from build123d import *

# Parameters (mm, degrees)
SKETCH_1_R               = 15.5
EXTRUDE_1_DEPTH          = 10
SKETCH_2_W               = 1.7
SKETCH_2_H               = 2.2
SKETCH_4_R               = 11.5
CUT_EXTRUDE_1_DEPTH      = 14
SKETCH_5_R               = 5.25
CUT_EXTRUDE_2_DEPTH      = 15
CHAMFER_1_SIZE           = 2
CUT_EXTRUDE_START        = -2
SKETCH_6_R               = 11.5
SKETCH_6_R_2             = 5
CUT_EXTRUDE_3_DEPTH      = 2
CHAMFER_2_SIZE           = 2
SKETCH_8_R               = 1.5
CUT_EXTRUDE_4_DEPTH      = 10
PATTERN_CIRCULAR_1_COUNT = 4
SKETCH_7_W               = 1.5
SKETCH_7_H               = 8
CHAMFER_5_SIZE           = 1.5
CHAMFER_4_SIZE           = 0.5


with BuildPart() as part:
    # 草图1 → 凸台-拉伸1 (new, symmetric)
    with BuildSketch(Plane(origin=(0, 0, 0), x_dir=(1, 0, 0), z_dir=(0, 1, 0))):
        with Locations(Location((0, 0, 0), (0, 0, 270))):
            Circle(SKETCH_1_R)
    extrude(amount=EXTRUDE_1_DEPTH, both=True)

    # 草图2 → 切除-旋转1 (revolve, cut)
    with BuildSketch(Plane.XY, mode=Mode.PRIVATE) as cut_revolve_1_sk:
        with Locations((14.65, 7.3)):
            Rectangle(SKETCH_2_W, SKETCH_2_H)
    cut_revolve_1 = revolve(cut_revolve_1_sk.sketch.rotate(Axis((0, 8.4, 0), (0, -1, 0)), 90), axis=Axis((0, 8.4, 0), (0, -1, 0)), mode=Mode.SUBTRACT)

    # 镜向1: 切除-旋转1 across plane
    add(cut_revolve_1.mirror(Plane.ZX), mode=Mode.SUBTRACT)

    # 草图4 → 切除-拉伸1 (cut)
    with BuildSketch(Plane.XZ.offset(10)):
        with Locations(Location((0, 0, 0), (0, 0, 270))):
            Circle(SKETCH_4_R)
    extrude(amount=-CUT_EXTRUDE_1_DEPTH, mode=Mode.SUBTRACT)

    # 草图5 → 切除-拉伸2 (cut)
    with BuildSketch(Plane(origin=(0, 10, 0), x_dir=(1, 0, 0), z_dir=(0, 1, 0))):
        with Locations(Location((0, 0, 0), (0, 0, 270))):
            Circle(SKETCH_5_R)
    extrude(amount=-CUT_EXTRUDE_2_DEPTH, mode=Mode.SUBTRACT)

    # 倒角1
    chamfer_1_edges = [part.edges().sort_by_distance(p)[0] for p in [
        (0, -10, 11.5),
    ]]
    chamfer(chamfer_1_edges, length=CHAMFER_1_SIZE)

    # 草图6 → 切除-拉伸3 (cut)
    with BuildSketch(Plane(origin=(0, 10, 0), x_dir=(1, 0, 0), z_dir=(0, 1, 0)).offset(CUT_EXTRUDE_START)):
        with Locations(Location((0, 0, 0), (0, 0, 90))):
            Circle(SKETCH_6_R)
        Circle(SKETCH_6_R_2, mode=Mode.SUBTRACT)
    extrude(amount=CUT_EXTRUDE_3_DEPTH, mode=Mode.SUBTRACT)

    # 倒角2
    chamfer_2_edges = [part.edges().sort_by_distance(p)[0] for p in [
        (0, 10, 11.5),
    ]]
    chamfer(chamfer_2_edges, length=CHAMFER_2_SIZE - 0.0001)  # a hair under: the kernel refuses the full size

    # 草图8 → 切除-拉伸4 (cut)
    with BuildSketch(Plane.XZ.offset(-4)):
        with Locations(Location((-8, 0, 0), (0, 0, 270))):
            Circle(SKETCH_8_R)
    cut_extrude_4 = extrude(amount=-CUT_EXTRUDE_4_DEPTH, mode=Mode.SUBTRACT)

    # 阵列(圆周)1: 切除-拉伸4 ×4 about axis
    pattern_circular_1_axis = Axis((0, 0, 0), (0, 1, 0))
    for i in range(1, PATTERN_CIRCULAR_1_COUNT):
        add(cut_extrude_4.rotate(pattern_circular_1_axis, i * 360 / PATTERN_CIRCULAR_1_COUNT), mode=Mode.SUBTRACT)

    # 草图7 → 切除-旋转2 (revolve, cut)
    with BuildSketch(Plane(origin=(0, 0, 0), x_dir=(0, 0, -1), z_dir=(1, 0, 0))):
        with Locations((14.75, 0)):
            Rectangle(SKETCH_7_W, SKETCH_7_H)
    revolve(axis=Axis((0, 4, 0), (0, 1, 0)), mode=Mode.SUBTRACT)

    # 倒角5
    chamfer_5_edges = [part.edges().sort_by_distance(p)[0] for p in [
        (0, -4, 14),
        (0, 4, 14),
    ]]
    chamfer(chamfer_5_edges, length=CHAMFER_5_SIZE - 0.0001)  # a hair under: the kernel refuses the full size

    # 倒角4
    chamfer_4_edges = [part.edges().sort_by_distance(p)[0] for p in [
        (0, 4, 11.5),
        (0, 4, -5.25),
        (0, 8, -5.25),
    ]]
    chamfer(chamfer_4_edges, length=CHAMFER_4_SIZE)


solid = part.part
Can you work these out from the model? Positions are in its coordinate system, mm. A direction names the side the tool comes from. Coordinates: 2 decimals unless noted, no trailing zeros. Order: outer loops, then holes, each group sorted by start corner. A loop starts at its lowest first (then second) coordinate and runs counter-clockwise, first axis right, second up. Notation, with made-up numbers: (81, -14.5) - (110, -14.5) arc R8 cw to (110, -10.5) - close; hole circle Ø8 at (-7.5, 29). An arc over 180 degrees is marked (long way). Answer as a JSON object with one key per item and string values. Group by question number.
Q1. Imagine slicing it at A-A (y = 7). Please give me the cut outline in (x, z), and give its area (3 significant figures).
Q2. On a 3-axis mill with a long thin cutter (end or side, diameter ignored), from which of +Z, -Z, +X, -X, +Y, -Y can I reach the whole of each face in a straight line? I mean faces 4 (the face through (9.7, -2.33, -6.18)), 5 (the face through (-2.7, 8, 5.3)), 6 (the face through (15.368, -9.189, -2.018)), 7 (the face through (1, -8.4, 14)). Say none if no direction works.
Q3. I need wall thicknesses on line 1 (X direction, y = 5.1, z = 0); line 2 (Y direction, x = 13, z = -6); line 3 (Y direction, x = -5, z = -9.5). Which ranges of each line are inside material? Lowest first, please. Write a range as from..to.
Q4. We'd pull the mould along Z, two halves only. Please class faces 1 (the face through (13, -10, -5)), 2 (the face through (1.6, 6, 5)), 3 (the face through (5.362, 0.035, -12.932)): +Z half, -Z half, draft (parallel to the pull), parting line (faces both ways), or undercut.
Q5. Will these pins go through, and if not, where does the flat tip stop? P1, Ø1.5, axis at y = -5, z = 1.5, coming from the -X side; P2, Ø18.5, axis at x = 3, z = 1, coming from the +Y side; P3, Ø5, axis at x = 0, z = -8, coming from the +Y side.
Q6. Imagine slicing it at D-D (y = -0.5). Please give me the cut outline in (x, z), and give its area (3 significant figures).
Q7. Imagine slicing it at B-B (x = 0). Give the number of separate pieces and of enclosed holes in the cut face, and give its area (3 significant figures).
Determined:
{
 "1": {"outline": "circle Ø27.6 at (0, 0); hole circle Ø3 at (-8, 0); hole circle Ø10.5 at (0, 0); hole circle Ø3 at (0, -8); hole circle Ø3 at (0, 8); hole circle Ø3 at (8, 0)", "area": "483 mm2"},
 "2": {"face 4": "-Y", "face 5": "+Y", "face 6": "+Y, -Y", "face 7": "none"},
 "3": {"line 1": "x = -15.5..-9.5, -6.5..-5.25, 5.25..6.5, 9.5..15.5", "line 2": "y = -10..-8.4, -6.2..-2.82, 2.82..6.2, 8.4..10", "line 3": "y = 4..8"},
 "4": {"face 1": "draft", "face 2": "undercut", "face 3": "parting line"},
 "5": {"P1": "stops at x = -15.48", "P2": "stops at y = 8.91", "P3": "stops at y = 8"},
 "6": {"outline": "circle Ø28 at (0, 0); hole circle Ø23 at (0, 0)", "area": "200 mm2"},
 "7": {"separate pieces": "4", "enclosed holes": "0", "area": "143 mm2"}
}
